Source: CAD feature listing. Evaluate the final solid. Frame: model axes, mm. Face numbers are marked on the shaded views. A direction names the side the tool comes from. Give positions to 0.01 mm unless a question says otherwise; leave off trailing zeros. Write each loop counter-clockwise with the first axis right and the second up, starting at its lowest first coordinate (ties: lowest second). Pieces come first, ordered by that corner, then holes. Notation, with made-up numbers: (-27.75, 50.5) -> (21.25, 50.5) arc R16 ccw to (21.25, 75.5) -> close; hole circle Ø9 at (86, -21). An arc over 180 degrees is marked (long way). Write item = value, one per line.
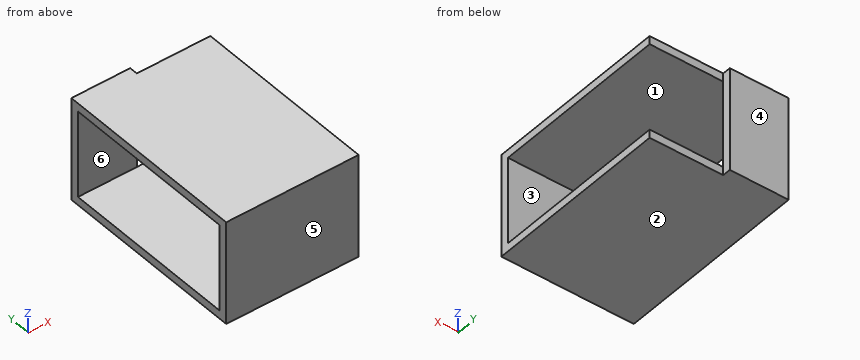
from build123d import *

# Parameters (mm, degrees)
SKETCH1_W           = 160
SKETCH1_H           = 215
BOSS_EXTRUDE1_DEPTH = 105
SHELL2_T            = 10
SKETCH6_W           = 88.9
SKETCH6_H           = 125
CUT_EXTRUDE3_DEPTH  = 10


with BuildPart() as part:
    # Sketch1 → Boss-Extrude1 (new body)
    with BuildSketch(Plane.XY):
        with Locations((80, 107.5)):
            Rectangle(SKETCH1_W, SKETCH1_H)
    extrude(amount=BOSS_EXTRUDE1_DEPTH)

    # Shell2
    shell2_openings = [part.faces().sort_by_distance(p)[0] for p in [
        (160, 107.5, 52.5),
        (0, 107.5, 52.5),
    ]]
    offset(amount=SHELL2_T, openings=shell2_openings, kind=Kind.INTERSECTION)

    # Sketch6 → Cut-Extrude3 (cut)
    with BuildSketch(Plane.XZ.offset(-225)):
        with Locations((115.55, 52.5)):
            Rectangle(SKETCH6_W, SKETCH6_H)
    extrude(amount=CUT_EXTRUDE3_DEPTH, mode=Mode.SUBTRACT)


solid = part.part
1) Material intervals for L1, parallel to Z at x = 45.5, y = 94; L2, parallel to Y at x = 50.5, z = 65.5; L3, parallel to Y at x = 137, z = 53.5, sorted ascending.
Computed:
L1 = -10 to 0, 105 to 115
L2 = -10 to 0, 215 to 225
L3 = -10 to 0
2) Access query for the marked faces 1 and 2. Directions: +Z, -Z, +X, -X, +Y, -Y. A direction counts if a zero-diameter tool reaches every point of the face in a straight line with its end or side. Return the directions, or none.
Computed:
face_1 = +X, -X
face_2 = -Z, +X, -X, +Y, -Y
3) Draft query along Y for the marked faces 3, 4, 5 and 6. Return one class per face: pulls with the +Y half, pulls with the -Y half, needs draft (parallel to the pull), parting line crosses it, or undercut.
Computed:
face_3 = undercut
face_4 = pulls with the +Y half
face_5 = pulls with the -Y half
face_6 = undercut
4) Cut plane B-B (x = 27.5). Return the cut outline in (y, z).
Computed:
outline = (-10, -10) -> (225, -10) -> (225, 115) -> (-10, 115) -> close; hole (0, 0) -> (215, 0) -> (215, 105) -> (0, 105) -> close
5) Cut plane C-C (z = 35). Return the cut outline in (x, y), then the cut area to 3 significant figures.
Computed:
outline = (0, -10) -> (160, -10) -> (160, 0) -> (0, 0) -> close; (0, 215) -> (71.1, 215) -> (71.1, 225) -> (0, 225) -> close
area = 2,310 mm²
6) Contact query for flat-ended pins moving along their axis: pin 1 (5 mm diameter, centred on x = 130, z = -5, fed in from +Y); pin 2 (1.5 mm diameter, centred on x = 125.5, z = 8, fed in from +Y); pin 3 (3 mm diameter, centred on y = 218, z = 80.5, fed in from +X). Output: stop coordinate, or through.
Computed:
pin_1 = 215
pin_2 = 0
pin_3 = 71.1
7) Cut plane D-D (x = 88.5). Return the cut outline in (y, z), then the cut area to 3 significant figures.
Computed:
outline = (-10, -10) -> (215, -10) -> (215, 0) -> (0, 0) -> (0, 105) -> (215, 105) -> (215, 115) -> (-10, 115) -> close
area = 5,550 mm²
8) Cut plane A-A (y = 146.5). Return the cut outline in (x, z).
Computed:
outline = (0, -10) -> (160, -10) -> (160, 0) -> (0, 0) -> close; (0, 105) -> (160, 105) -> (160, 115) -> (0, 115) -> close
